Autodesk Inventor part; units mm, degrees
ref_plane "YZ Plane" through (0, 0, 0) normal (1, 0, 0) x (0, 1, 0)
ref_plane "XZ Plane" through (0, 0, 0) normal (0, 1, 0) x (-1, 0, 0)
ref_plane "XY Plane" through (0, 0, 0) normal (0, 0, 1) x (1, 0, 0)
sketch "Sketch1" plane through (0, 0, 0) normal (0, 0, 1) x (1, 0, 0)
  line L0 (-110, 70) -> (110, 70) construction
  line L1 (110, 70) -> (110, -70) construction
  line L2 (110, -70) -> (-110, -70) construction
  line L3 (-110, -70) -> (-110, 70) construction
  circle A0 centre (-90, 55) radius 5
  circle A1 centre (-90, -55) radius 5
  circle A2 centre (90, -55) radius 5
  circle A3 centre (-10, 45) radius 5
  line L4 (-67, 0) -> (-42, 0) construction
  line L5 (-42, 0) -> (-42, -30) construction
  line L6 (-42, -30) -> (-67, -30) construction
  line L7 (-67, -30) -> (-67, 0) construction
  circle A4 centre (-54.5, -11) radius 10 construction
  circle A5 centre (-63.5044, -24.4163) radius 3 construction
  circle A6 centre (-57.3559, -26.4695) radius 3 construction
  circle A7 centre (-51.263, -24.6531) radius 3 construction
  circle A8 centre (-45.3418, -26.5938) radius 3 construction
  arc A9 (-80.8676, 50.9258) -> (-100, 55) centre (-90, 55) ccw
  arc A10 (-4.8937, 53.598) -> (-15.7422, 53.187) centre (-10, 45) ccw
  arc A11 (90.4874, -64.9881) -> (88.2039, -45.1626) centre (90, -55) ccw
  line L8 (-100, 55) -> (-102.0827, 28.5336) construction
  line L9 (-102.0827, 28.5336) -> (-102.0827, 6.1317) construction
  line L10 (-102.0827, 6.1317) -> (-102.0827, -9.3012) construction
  line L11 (-102.0827, -9.3012) -> (-100, -55) construction
  spline S0 degree 4 poles (-100, 55) (-102.0827, 28.5336) (-102.0827, 6.1317) (-102.0827, -9.3012) (-100, -55) knots 1 1 1 1 1 2 2 2 2 2
  line L12 (-80.5098, 51.8478) -> (-81.3111, 50.3761) construction
  line L13 (-33.5621, 40.6884) -> (-15.7422, 53.187) construction
  spline S1 degree 3 poles (-74.3051, 13.1026) (-63.5044, 21.906) (-33.5621, 40.6884) (-15.7422, 53.187) knots 1.047287 1.047287 1.047287 1.047287 2 2 2 2
  line L14 (-90, -65) -> (-53.427, -70) construction
  line L15 (-53.427, -70) -> (0, -70) construction
  line L16 (0, -70) -> (41.9992, -67.3543) construction
  line L17 (41.9992, -67.3543) -> (90.4874, -64.9881) construction
  spline S2 degree 4 poles (-90, -65) (-53.427, -70) (0, -70) (41.9992, -67.3543) (90.4874, -64.9881) knots 1 1 1 1 1 2 2 2 2 2
  arc A12 (-100, -55) -> (-90, -65) centre (-90, -55) ccw
  spline S3 degree 3 poles (-86.2173, -25.9445) (-74.5546, -4.3329) (-47.6722, 13.3107) (-14.3115, 31.1686) knots 1.116691 1.116691 1.116691 1.116691 1.90623 1.90623 1.90623 1.90623
  line L18 (-86.2173, -25.9445) -> (-74.5546, -4.3329) construction
  spline S4 degree 4 poles (-80.5098, 51.8478) (-81.3111, 50.3761) (-83.3432, 41.5365) (-84.547, 29.8741) (-86.4048, 20.3523) knots 1 1 1 1 1 1.500456 1.500456 1.500456 1.500456 1.500456
  spline S5 degree 4 poles (-86.2173, -25.9445) (-87.4499, -31.1305) (-87.0929, -33.8364) (-86.699, -36.6544) (-86.2648, -39.5964) knots 1.850189 1.850189 1.850189 1.850189 1.850189 1.936877 1.936877 1.936877 1.936877 1.936877
  line L19 (-86.2173, -25.9445) -> (-87.4499, -31.1305) construction
  arc A13 (-86.2648, -39.5964) -> (-80.2389, -45.8706) centre (-78.8452, -38.5013) ccw
  line L20 (-87.4499, -31.1305) -> (-87.0929, -33.8364) construction
  line L21 (-87.0929, -33.8364) -> (-86.699, -36.6544) construction
  line L22 (-86.699, -36.6544) -> (-86.2648, -39.5964) construction
  arc A14 (-86.4048, 20.3523) -> (-74.3051, 13.1026) centre (-79.0436, 18.9161) ccw
  line L23 (-81.3111, 50.3761) -> (-83.3432, 41.5365) construction
  line L24 (-83.3432, 41.5365) -> (-84.547, 29.8741) construction
  line L25 (-84.547, 29.8741) -> (-86.4048, 20.3523) construction
  line L26 (-74.3051, 13.1026) -> (-63.5044, 21.906) construction
  line L27 (-63.5044, 21.906) -> (-33.5621, 40.6884) construction
  spline S6 degree 4 poles (-6.0641, 29.79) (10.6281, 14.0219) (25.4029, -2.497) (40.3618, -18.7245) (53.6143, -31.8741) knots 1.041568 1.041568 1.041568 1.041568 1.041568 1.754128 1.754128 1.754128 1.754128 1.754128
  line L28 (-4.8937, 53.598) -> (11.2306, 41.5365) construction
  line L29 (11.2306, 41.5365) -> (41.9992, 15.4144) construction
  line L30 (41.9992, 15.4144) -> (73.02, -16.6008) construction
  line L31 (73.02, -16.6008) -> (98.2566, -49.3583) construction
  spline S7 degree 4 poles (-4.8937, 53.598) (11.2306, 41.5365) (41.9992, 15.4144) (73.02, -16.6008) (98.2566, -49.3583) knots 1 1 1 1 1 2 2 2 2 2
  line L32 (-80.2389, -45.8706) -> (-53.343, -43.1999) construction
  line L33 (-53.343, -43.1999) -> (-23.1335, -44.327) construction
  spline S8 degree 4 poles (-80.2389, -45.8706) (-53.343, -43.1999) (-23.1335, -44.327) (4.8754, -43.9641) (34.4585, -44.2782) (48.1029, -44.6945) knots 1 1 1 1 1 2 2.688212 2.688212 2.688212 2.688212 2.688212
  arc A15 (48.1029, -44.6945) -> (53.6143, -31.8741) centre (48.3317, -37.198) ccw
  line L34 (40.3618, -18.7245) -> (53.6143, -31.8741) construction
  line L35 (-23.1335, -44.327) -> (4.8754, -43.9641) construction
  line L36 (4.8754, -43.9641) -> (34.4585, -44.2782) construction
  line L37 (34.4585, -44.2782) -> (48.1029, -44.6945) construction
  arc A16 (-6.0641, 29.79) -> (-15.1895, 30.6979) centre (-11.2144, 24.338) ccw
  line L38 (-74.5546, -4.3329) -> (-47.6722, 13.3107) construction
  line L39 (-47.6722, 13.3107) -> (-14.3115, 31.1686) construction
  line L40 (-6.0641, 29.79) -> (10.6281, 14.0219) construction
  line L41 (10.6281, 14.0219) -> (25.4029, -2.497) construction
  line L42 (25.4029, -2.497) -> (40.3618, -18.7245) construction
  point P0 (0, 0)
  dimension "d1" = 70
  dimension "d2" = 70
  dimension "d3" = 110
  dimension "d4" = 110
  dimension "d5" = 10
  dimension "d6" = 10
  dimension "d7" = 10
  dimension "d8" = 10
  dimension "d9" = 55
  dimension "d10" = 55
  dimension "d11" = 55
  dimension "d12" = 180
  dimension "d13" = 90
  dimension "d14" = 90
  dimension "d15" = 10
  dimension "d16" = 45
  dimension "d17" = 42
  dimension "d18" = 30
  dimension "d19" = 0
  dimension "d20" = 25
  dimension "d21" = 20
  dimension "d22" = 6
  dimension "d23" = 6
  dimension "d24" = 6
  dimension "d25" = 11
  dimension "d26" = 12.5
  dimension "d27" = 6
  dimension "d28" = 20
  dimension "d29" = 20
  dimension "d30" = 20
  dimension "d37" = 15
  dimension "d38" = 15
  dimension "d41" = 15
  dimension "d42" = 15
extrude "Extrusion3" add sketch "Sketch1" along normal blind 9.4 contours S4 A14 S1 A10 S7 A11 S2 A12 S0 A9
equation "\"d26\" = 0.5 * d20"
properties part number "Bracket Concept MK2"
Source: CAD feature listing. Evaluate the final solid. Frame: model axes, mm. A direction names the side the tool comes from. Give positions to 0.01 mm unless a question says otherwise; leave off trailing zeros. Order: outer loops, then holes, each group sorted by start corner. A loop starts at its lowest first (then second) coordinate and runs counter-clockwise, first axis right, second up. Notation, with made-up numbers: (-13, 53.5) -> (38, 53.5) arc R29 cw to (38, 84.5) -> close; hole circle Ø2 at (-7.5, 16). An arc over 180 degrees is marked (long way). Write item = value, one per line.
Item 1: Section query B-B (x = -10). State how many separate pieces and enclosed holes the cut face has, then the cut area to 3 significant figures.
Check result:
separate_pieces = 3
enclosed_holes = 0
area = 357 mm²
Item 2: Ray query, probe 1 along Y at (x, z) = (-90, 7); probe 2 along X at (y, z) = (23, 4); probe 3 along X at (y, z) = (40.5, 5.5). Return the intervals inside material, ascending.
Check result:
probe_1 = -65 to -60, -50 to 50, 60 to 65
probe_2 = -101.63 to -85.92, -60.67 to -29.09, 0.95 to 31.29
probe_3 = -100.95 to -83.09, -34.48 to -12.18, -7.82 to 11.47
Item 3: Set-up query: faces 4 (the face through (-96.99, -62.15, 4.63)), 5 (the face through (-84.21, -43.74, 4.63)). Return all of +Z, -Z, +X, -X, +Y, -Y with unobstructed straight access to the full face (end or side cutting, diameter ignored); none if empty.
Check result:
face_4 = +Z, -Z, -X, -Y
face_5 = +Z, -Z
Item 4: Section query A-A (y = -58). Output: boundary loops of the cut face in (x, z), then the cut area to 3 significant figures.
Check result:
outline = (-99.54, 0) -> (-94, 0) -> (-94, 9.4) -> (-99.54, 9.4) -> close; (-86, 0) -> (86, 0) -> (86, 9.4) -> (-86, 9.4) -> close; (94, 0) -> (99.54, 0) -> (99.54, 9.4) -> (94, 9.4) -> close
area = 1,720 mm²
Item 5: Mould query, pull axis Y, two halves, no side actions, for faces 1 (the face through (93, -59, 5)), 2 (the face through (-25, -47, 0)), 3 (the face through (-10, 55, 5)). Classes: +Y half, -Y half, draft (parallel to the pull), parting line (faces both ways), or undercut.
Check result:
face_1 = undercut
face_2 = draft
face_3 = +Y half
Item 6: Contact query for a flat-ended pin moving along its axis: pin 1 (2 mm diameter, centred on x = -43, y = 29.5, fed in from -Z). Output: stop coordinate, or through.
Check result:
pin_1 = 0
